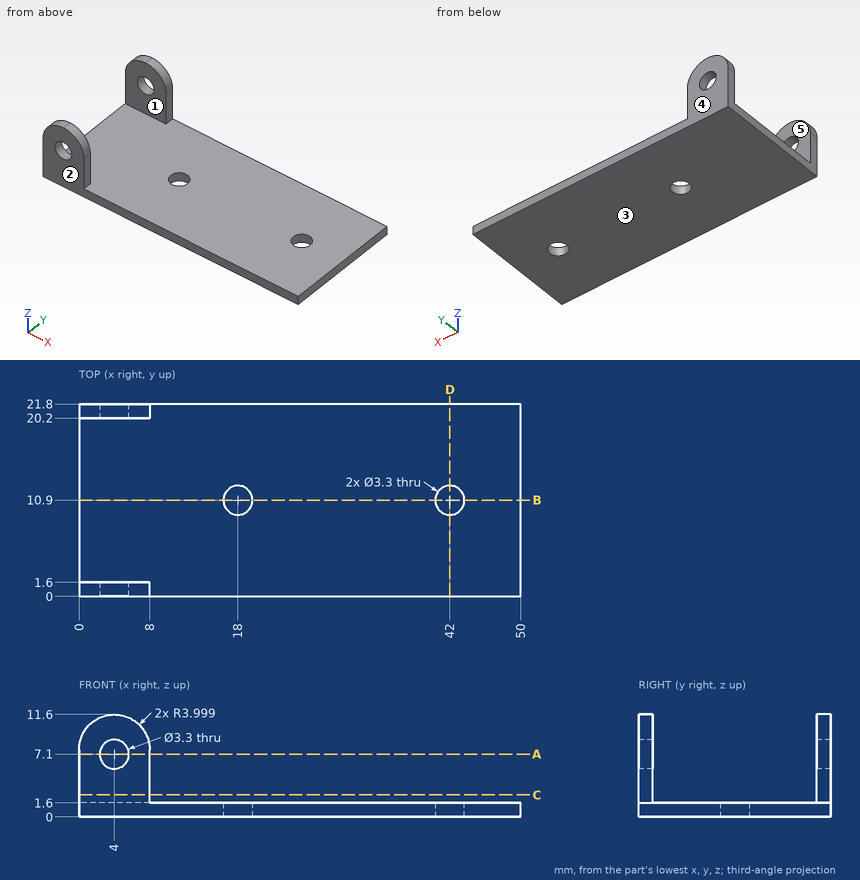
Answer from the drawing. Dimensions are ordinates in mm from the lowest x, y and z of the part. A direction names the side the tool comes from. Coordinates: 2 decimals unless noted, no trailing zeros. Loops run counter-clockwise (first coordinate to the right, second up) from the corner with the lowest first, then second, coordinate; pieces in that order, holes last. Notation, with made-up numbers: (-15.75, -33.5) - (34.25, -33.5) arc R11 ccw to (34.25, -25.5) - close; hole circle Ø10 at (78, 52.25). An arc over 180 degrees is marked (long way). Use a Markdown table: item, result.
Item 1: Find section C-C, the plane z = 2.5. Determine the outline of the cut face in (x, y), and give its area (3 significant figures).
Evaluation:
| item | result |
|---|---|
| outline | (0, 0) - (8, 0) - (8, 1.6) - (0, 1.6) - close; (0, 20.2) - (8, 20.2) - (8, 21.8) - (0, 21.8) - close |
| area | 25.6 mm2 |
Item 2: Consider probe 1 along Z at (x, y) = (4, 1.1); probe 2 along Y at (x, z) = (4, 3.25); probe 3 along Y at (x, z) = (18, 0.9). Determine where each line is inside the solid, lowest interval first. Write a range as from..to.
Evaluation:
| item | result |
|---|---|
| probe 1 | z = 0..5.45, 8.75..11.6 |
| probe 2 | y = 0..1.6, 20.2..21.8 |
| probe 3 | y = 0..9.25, 12.55..21.8 |
Item 3: For the marked faces 1 and 2, determine the directions among +Z, -Z, +X, -X, +Y, -Y from which every point of the face is accessible in a straight line to the end or side of a thin tool.
Evaluation:
| item | result |
|---|---|
| face 1 | +Z, +X, -X |
| face 2 | +Z, -Z, +X, -X, -Y |
Item 4: Given pin 1 Ø0.8 at (y, z) = (1, 4.5) entering from +X; pin 2 Ø6 at (x, y) = (31.5, 14) entering from +Z, each flat-ended and moving along its own axis, determine where each tip first touches the part or whether it passes through.
Evaluation:
| item | result |
|---|---|
| pin 1 | stops at x = 8 |
| pin 2 | stops at z = 1.6 |
Item 5: Find section A-A, the plane z = 7.1. Determine the outline of the cut face in (x, y).
Evaluation:
| item | result |
|---|---|
| outline | (0, 0) - (2.35, 0) - (2.35, 1.6) - (0, 1.6) - close; (0, 20.2) - (2.35, 20.2) - (2.35, 21.8) - (0, 21.8) - close; (5.65, 0) - (8, 0) - (8, 1.6) - (5.65, 1.6) - close; (5.65, 20.2) - (8, 20.2) - (8, 21.8) - (5.65, 21.8) - close |
Item 6: The mould has two halves that part along Y. Classify the marked faces 3, 4 and 5: +Y half, -Y half, draft (parallel to the pull), parting line (faces both ways), or undercut.
Evaluation:
| item | result |
|---|---|
| face 3 | draft |
| face 4 | +Y half |
| face 5 | undercut |
Item 7: Find section D-D, the plane x = 42. Determine the outline of the cut face in (y, z).
Evaluation:
| item | result |
|---|---|
| outline | (0, 0) - (9.25, 0) - (9.25, 1.6) - (0, 1.6) - close; (12.55, 0) - (21.8, 0) - (21.8, 1.6) - (12.55, 1.6) - close |
Item 8: Find section B-B, the plane y = 10.9. Determine the outline of the cut face in (x, z).
Evaluation:
| item | result |
|---|---|
| outline | (0, 0) - (16.35, 0) - (16.35, 1.6) - (0, 1.6) - close; (19.65, 0) - (40.35, 0) - (40.35, 1.6) - (19.65, 1.6) - close; (43.65, 0) - (50, 0) - (50, 1.6) - (43.65, 1.6) - close |
